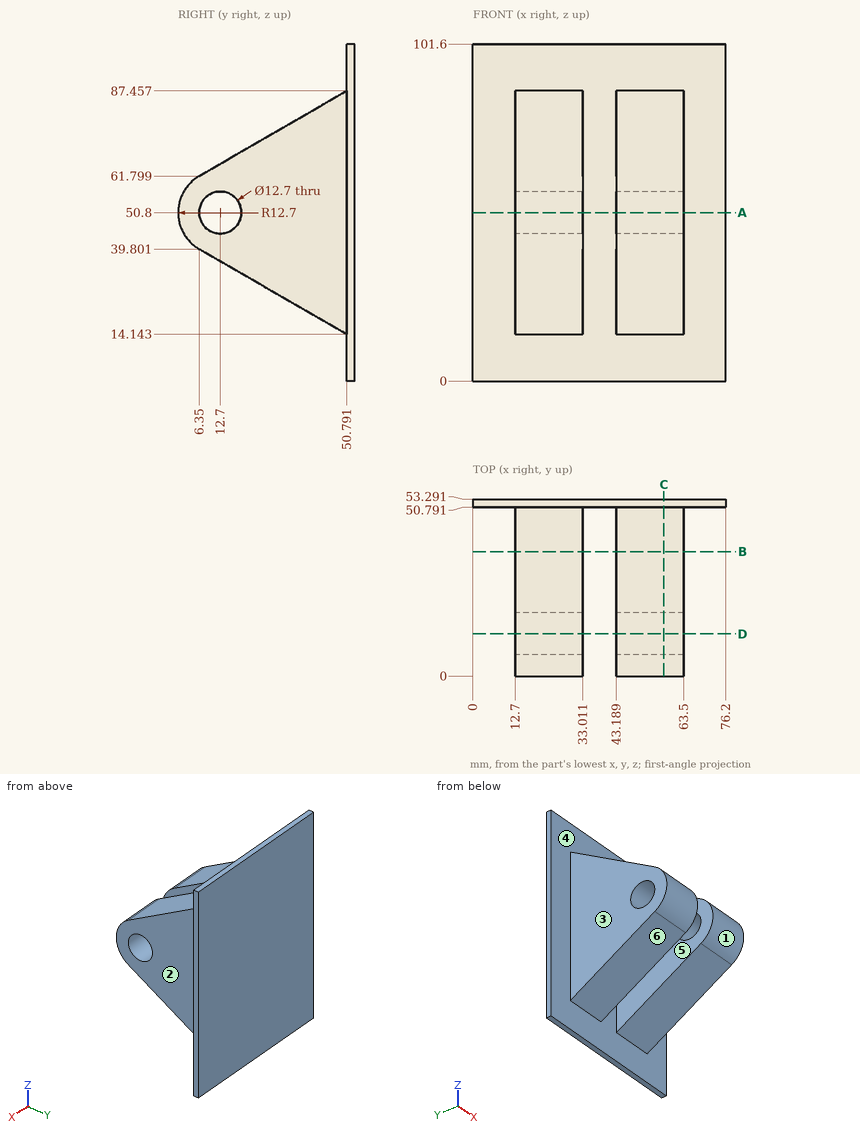
Source: three-view drawing plus pictorial views. Frame: mm from the lowest corner of the part. A direction names the side the tool comes from. Round coordinates to 2 decimals unless told otherwise and drop trailing zeros. Loops run counter-clockwise (first coordinate to the right, second up) from the corner with the lowest first, then second, coordinate; pieces in that order, holes last.
Q1. Section D-D, the plane y = 12.7. State how many separate pieces and enclosed holes the cut face has.
Q2. Section A-A, the plane z = 50.8. Return loops of the section in (x, y).
Q3. Access query for the marked faces 5 and 6. Directions: +Z, -Z, +X, -X, +Y, -Y. A direction counts if a zero-diameter tool reaches every point of the face in a straight line with its end or side. Return the directions, or none.
Q4. Section B-B, the plane y = 37.5. Return loops of the section in (x, z).
Q5. Section C-C, the plane x = 57.5. Return loops of the section in (y, z), plus the area to 3 significant figures.
Q6. Ray query, line 1 (X direction, y = 28.5, z = 40); line 2 (Y direction, x = 49, z = 50.8); line 3 (Z direction, x = 17, y = 12). Return the intervals inside material, ascending.
Q7. First-contact query: P1, Ø8, axis at x = 35.5, y = 32, coming from the +Z side (1 decimal); P2, Ø1, axis at x = 56.5, y = 16.5, coming from the -Z side; P3, Ø1, axis at x = 28, z = 57.5, coming from the -Y side (1 decimal). Flat tips, straight axial feed; report the tip coordinate or a pass-through.
Q8. Mould query, pull axis X, two halves, no side actions, for the marked faces 1, 2, 3 and 4. Classes: pulls with the +X half, pulls with the -X half, needs draft (parallel to the pull), parting line crosses it, or undercut.
Solutions:
1. separate pieces: 4
1. enclosed holes: 0
2. outline: (0, 50.79) - (12.7, 50.79) - (12.7, 19.05) - (33.01, 19.05) - (33.01, 50.79) - (43.19, 50.79) - (43.19, 19.05) - (63.5, 19.05) - (63.5, 50.79) - (76.2, 50.79) - (76.2, 53.29) - (0, 53.29) - close; (12.7, 0) - (33.01, 0) - (33.01, 6.35) - (12.7, 6.35) - close; (43.19, 0) - (63.5, 0) - (63.5, 6.35) - (43.19, 6.35) - close
3. face 5: +Z, -Z, -Y
3. face 6: -Z, +X, -X, -Y
4. outline: (12.7, 21.82) - (33.01, 21.82) - (33.01, 79.78) - (12.7, 79.78) - close; (43.19, 21.82) - (63.5, 21.82) - (63.5, 79.78) - (43.19, 79.78) - close
5. outline: (6.35, 39.8) - (50.79, 14.14) - (50.79, 0) - (53.29, 0) - (53.29, 101.6) - (50.79, 101.6) - (50.79, 87.46) - (6.35, 61.8) arc R12.7 ccw to start; hole circle Ø12.7 at (12.7, 50.8)
5. area: 2,340 mm2
6. line 1: x = 12.7 to 33.01, 43.19 to 63.5
6. line 2: y = 0 to 6.35, 19.05 to 53.29
6. line 3: z = 36.54 to 44.49, 57.11 to 65.06
7. P1: stops at z = 78.4
7. P2: stops at z = 33.65
7. P3: stops at y = 1.6
8. face 1: needs draft
8. face 2: pulls with the +X half
8. face 3: pulls with the -X half
8. face 4: undercut
